from build123d import *

# Parameters (mm, degrees)
BOSS_EXTRUDE2_DEPTH                            = 4
SKETCH2_R                                      = 5
CUT_EXTRUDE1_DEPTH                             = 107.141415103
CSK_FOR_M4_FLAT_HEAD_MACHINE_SCREW2_AT_2_COUNT = 2
CSK_FOR_M4_FLAT_HEAD_MACHINE_SCREW2_AT_2_PITCH = 12
CHAMFER1_SIZE                                  = 4


with BuildPart() as part:
    # Sketch1 → Boss-Extrude2 (new body)
    with BuildSketch(Plane(origin=(0, 0, 0), x_dir=(1, 0, 0), z_dir=(0, 1, 0))):
        Polygon((-75, 75), (-75, -75), (-67, -75), (67, -75), (75, -75), (75, 75), (67, 75), (-67, 75), align=None)
        with BuildLine():
            ThreePointArc((-22.004968974, 33.403313316), (0, 40), (22.004968974, 33.403313316))
            ThreePointArc((22.004968974, 33.403313316), (22.894438748, 31.935685036), (22.318934087, 30.318934087))
            Line((22.318934087, 30.318934087), (4.949747468, 12.949747468))
            ThreePointArc((4.949747468, 12.949747468), (0, 10.899494937), (-4.949747468, 12.949747468))
            Line((-4.949747468, 12.949747468), (-22.318934087, 30.318934087))
            ThreePointArc((-22.318934087, 30.318934087), (-22.894438748, 31.935685036), (-22.004968974, 33.403313316))
        make_face(mode=Mode.SUBTRACT)
        with BuildLine():
            Line((8, -5.514718626), (8, 5.514718626))
            ThreePointArc((8, 5.514718626), (8.456722805, 7.81081922), (9.757359313, 9.757359313))
            Line((9.757359313, 9.757359313), (55.050252532, 55.050252532))
            ThreePointArc((55.050252532, 55.050252532), (62.678784027, 56.567661791), (67, 50.100505063))
            Line((67, 50.100505063), (67, -50.100505063))
            ThreePointArc((67, -50.100505063), (62.678784027, -56.567661791), (55.050252532, -55.050252532))
            Line((55.050252532, -55.050252532), (9.757359313, -9.757359313))
            ThreePointArc((9.757359313, -9.757359313), (8.456722805, -7.81081922), (8, -5.514718626))
        make_face(mode=Mode.SUBTRACT)
        with BuildLine():
            Line((-16, -67), (-59, -67))
            Line((-59, -67), (-33.568239019, -41.568239019))
            ThreePointArc((-33.568239019, -41.568239019), (-31.098923321, -40.412818885), (-28.462788791, -41.108024207))
            ThreePointArc((-28.462788791, -41.108024207), (-20.569707054, -45.572877369), (-12, -48.538644398))
            Line((-12, -48.538644398), (-12, -63))
            ThreePointArc((-12, -63), (-13.171572875, -65.828427125), (-16, -67))
        make_face(mode=Mode.SUBTRACT)
        with BuildLine():
            Line((33.568239019, -41.568239019), (59, -67))
            Line((59, -67), (16, -67))
            ThreePointArc((16, -67), (13.171572875, -65.828427125), (12, -63))
            Line((12, -63), (12, -48.538644398))
            ThreePointArc((12, -48.538644398), (20.569707054, -45.572877369), (28.462788791, -41.108024207))
            ThreePointArc((28.462788791, -41.108024207), (31.098923321, -40.412818885), (33.568239019, -41.568239019))
        make_face(mode=Mode.SUBTRACT)
        with BuildLine():
            ThreePointArc((-4.949747468, -12.949747468), (0, -10.899494937), (4.949747468, -12.949747468))
            Line((4.949747468, -12.949747468), (22.318934087, -30.318934087))
            ThreePointArc((22.318934087, -30.318934087), (22.894438748, -31.935685036), (22.004968974, -33.403313316))
            ThreePointArc((22.004968974, -33.403313316), (0, -40), (-22.004968974, -33.403313316))
            ThreePointArc((-22.004968974, -33.403313316), (-22.894438748, -31.935685036), (-22.318934087, -30.318934087))
            Line((-22.318934087, -30.318934087), (-4.949747468, -12.949747468))
        make_face(mode=Mode.SUBTRACT)
        with BuildLine():
            Line((-67, -50.100505063), (-67, 50.100505063))
            ThreePointArc((-67, 50.100505063), (-62.678784027, 56.567661791), (-55.050252532, 55.050252532))
            Line((-55.050252532, 55.050252532), (-9.757359313, 9.757359313))
            ThreePointArc((-9.757359313, 9.757359313), (-8.456722805, 7.81081922), (-8, 5.514718626))
            Line((-8, 5.514718626), (-8, -5.514718626))
            ThreePointArc((-8, -5.514718626), (-8.456722805, -7.81081922), (-9.757359313, -9.757359313))
            Line((-9.757359313, -9.757359313), (-55.050252532, -55.050252532))
            ThreePointArc((-55.050252532, -55.050252532), (-62.678784027, -56.567661791), (-67, -50.100505063))
        make_face(mode=Mode.SUBTRACT)
        with BuildLine():
            Line((-33.568239019, 41.568239019), (-59, 67))
            Line((-59, 67), (-16, 67))
            ThreePointArc((-16, 67), (-13.171572875, 65.828427125), (-12, 63))
            Line((-12, 63), (-12, 48.538644398))
            ThreePointArc((-12, 48.538644398), (-20.569707054, 45.572877369), (-28.462788791, 41.108024207))
            ThreePointArc((-28.462788791, 41.108024207), (-31.098923321, 40.412818885), (-33.568239019, 41.568239019))
        make_face(mode=Mode.SUBTRACT)
        with BuildLine():
            Line((59, 67), (33.568239019, 41.568239019))
            ThreePointArc((33.568239019, 41.568239019), (31.098923321, 40.412818885), (28.462788791, 41.108024207))
            ThreePointArc((28.462788791, 41.108024207), (20.569707054, 45.572877369), (12, 48.538644398))
            Line((12, 48.538644398), (12, 63))
            ThreePointArc((12, 63), (13.171572875, 65.828427125), (16, 67))
            Line((16, 67), (59, 67))
        make_face(mode=Mode.SUBTRACT)
    extrude(amount=BOSS_EXTRUDE2_DEPTH)

    # Sketch2 → Cut-Extrude1 (cut, through all)
    with BuildSketch(Plane(origin=(0, 4, 0), x_dir=(1, 0, 0), z_dir=(0, 1, 0))):
        with Locations(Location((0, 0, 0), (0, 0, 270))):
            Circle(SKETCH2_R)
    extrude(amount=-CUT_EXTRUDE1_DEPTH, mode=Mode.SUBTRACT)

    # Sketch4 → CSK for M4 Flat Head Machine Screw1 (revolve, cut)
    with BuildSketch(Plane(origin=(-62.687827406, 4, -62.687827406), x_dir=(0, 0, 1), z_dir=(1, 0, 0))):
        Polygon((0, 0), (0, 4), (2.25, 4), (2.25, 2.45), (4.7, 0), align=None)
    csk_for_m4_flat_head_machine_screw1 = revolve(axis=Axis((-62.687827406, 10.35, -62.687827406), (0, -1, 0)), mode=Mode.SUBTRACT)

    # Mirror1: CSK for M4 Flat Head Machine Screw1 across plane
    add(csk_for_m4_flat_head_machine_screw1.mirror(Plane.XY), mode=Mode.SUBTRACT)

    # Mirror1 at the second plane: CSK for M4 Flat Head Machine Screw1 across plane
    add(csk_for_m4_flat_head_machine_screw1.mirror(Plane(origin=(0, 0, 0), x_dir=(0, 0, 1), z_dir=(1, 0, 0))), mode=Mode.SUBTRACT)

    # Mirror1 at the second plane copy 1 sketc → Mirror1 at the second plane copy 1 (revolve, cut)
    with BuildSketch(Plane(origin=(62.687827406, 4, 62.687827406), x_dir=(0, 0, -1), z_dir=(-1, 0, 0))):
        Polygon((0, 0), (0, 4), (2.25, 4), (2.25, 2.45), (4.7, 0), align=None)
    revolve(axis=Axis((62.687827406, 10.35, 62.687827406), (0, -1, 0)), mode=Mode.SUBTRACT)

    # Sketch10 → CSK for M4 Flat Head Machine Screw2 (revolve, cut)
    with BuildSketch(Plane(origin=(6, 4, -62.3846611), x_dir=(0, 0, 1), z_dir=(1, 0, 0))):
        Polygon((0, 0), (0, 4), (2.25, 4), (2.25, 2.45), (4.7, 0), align=None)
    csk_for_m4_flat_head_machine_screw2 = revolve(axis=Axis((6, 10.35, -62.3846611), (0, -1, 0)), mode=Mode.SUBTRACT)

    # CSK for M4 Flat Head Machine Screw2 at 2: CSK for M4 Flat Head Machine Screw2 ×2
    with Locations(*[(-i * CSK_FOR_M4_FLAT_HEAD_MACHINE_SCREW2_AT_2_PITCH, 0, 0) for i in range(1, CSK_FOR_M4_FLAT_HEAD_MACHINE_SCREW2_AT_2_COUNT)]):
        add(csk_for_m4_flat_head_machine_screw2, mode=Mode.SUBTRACT)

    # Mirror2: CSK for M4 Flat Head Machine Screw2 across plane
    add(csk_for_m4_flat_head_machine_screw2.mirror(Plane.XY), mode=Mode.SUBTRACT)

    # Mirror2 copy 1 sketch → Mirror2 copy 1 (revolve, cut)
    with BuildSketch(Plane(origin=(-6, 4, 62.3846611), x_dir=(0, 0, -1), z_dir=(1, 0, 0))):
        Polygon((0, 0), (0, -4), (2.25, -4), (2.25, -2.45), (4.7, 0), align=None)
    revolve(axis=Axis((-6, 10.35, 62.3846611), (0, 1, 0)), mode=Mode.SUBTRACT)

    # Chamfer1
    chamfer1_edges = [part.edges().sort_by_distance(p)[0] for p in [
        (0, 0, -75),
        (-75, 0, 0),
        (0, 0, 75),
        (75, 0, 0),
    ]]
    chamfer(chamfer1_edges, length=CHAMFER1_SIZE - 0.0001)  # a hair under: the kernel refuses the full size


solid = part.part
Verification items for the finished model (mm, model axes). A direction names the side the tool comes from. Round coordinates to 2 decimals unless told otherwise and drop trailing zeros. Use one line per item in the form item = value.
1. Access from +Z, -Z, +X, -X, +Y, -Y to the whole of each face (thin tool, end or side, straight path). Record for faces 3 (the conical face through (-60.56, 1.7, -61.58)), 4 (the cylindrical face through (-62.79, 1.97, -56.52)).
A:
face_3 = +Y
face_4 = +Y, -Y
2. Gauge pin test, flat ends, axial feed: pin 1 Ø5 at (x, z) = (62.69, 62.69) entering from +Y; pin 2 Ø5 at (x, z) = (6, 62.38) entering from -Y; pin 3 Ø1.2 at (y, z) = (2.5, 0.5) entering from -X; pin 4 Ø1.2 at (y, z) = (2.5, -1.5) entering from +X. Record the tip position at first contact, or that the pin passes through.
A:
pin_1 = 1.8
pin_2 = 0
pin_3 = -74.1
pin_4 = 74.1
3. Draft check along Z on faces 1 (the flat face through (0, 0, -6)), 2 (the conical face through (-60.56, 1.7, 61.58)). Enter one of: pulls with the +Z half, pulls with the -Z half, needs draft (parallel to the pull), parting line crosses it, or undercut.
A:
face_1 = needs draft
face_2 = undercut
4. Scan lines: probe 1 along Z at (x, y) = (-38, 2.7); probe 2 along Z at (x, y) = (-34.5, 0.95); probe 3 along X at (y, z) = (2.4, -24). Record each from-to range of solid material in increasing order.
A:
probe_1 = -73.7 to -67, -46 to -38, 38 to 46, 67 to 73.7
probe_2 = -71.95 to -67, -42.5 to -34.5, 34.5 to 42.5, 67 to 71.95
probe_3 = -73.4 to -67, -24 to -16, 16 to 24, 67 to 73.4
5. Section check A-A on z = 27. Give the number of separate pieces and of enclosed holes in the cut face, and give its area (3 significant figures).
A:
separate_pieces = 4
enclosed_holes = 0
area = 112 mm²
